Input: part model. Units: mm. Frame: model coordinates. Face numbers are marked on the shaded views. A direction names the side the tool comes from. Give positions to 0.01 mm unless a question says otherwise; leave off trailing zeros. Write each loop counter-clockwise with the first axis right and the second up, starting at its lowest first coordinate (ties: lowest second). Pieces come first, ordered by that corner, then holes. Notation, with made-up numbers: (-23.5, -36) - (-3.5, -36) arc R15 cw to (-3.5, -18) - close; hole circle Ø8 at (-2, 4.25). An arc over 180 degrees is marked (long way). Answer as CSV lines item,"result". Start each with the question number.
Autodesk Inventor part; units mm, degrees
ref_plane "YZ Plane" through (0, 0, 0) normal (1, 0, 0) x (0, 1, 0)
ref_plane "XZ Plane" through (0, 0, 0) normal (0, 1, 0) x (-1, 0, 0)
ref_plane "XY Plane" through (0, 0, 0) normal (0, 0, 1) x (1, 0, 0)
sketch "Sketch1" plane through (0, 0, 0) normal (0, 0, 1) x (1, 0, 0)
  arc A0 (-3.75, -2.5) -> (-3.75, -5) centre (-3.75, -3.75) ccw
  arc A1 (3.75, -5) -> (3.75, -2.5) centre (3.75, -3.75) ccw
  line L0 (-3.75, -2.5) -> (3.75, -2.5)
  line L1 (3.75, -5) -> (-3.75, -5)
  circle A2 centre (-3.75, -3.75) radius 0.75
  circle A3 centre (3.75, -3.75) radius 0.5
  circle A4 centre (3.75, -3.75) radius 0.5
  point P0 (0, 0)
  dimension "d0" = 2.5
  dimension "d1" = 5
  dimension "d4" = 7.5
  dimension "d5" = 3.75
  dimension "d6" = 1.5
  dimension "d7" = 1
  dimension "d77" = 1
extrude "Extrusion1" add sketch "Sketch1" along normal blind 20
sketch "Sketch3" plane through (0, 0, 0) normal (0, 1, 0) x (-1, 0, 0)
  line L0 (5, 0) -> (3.75, 0)
  line L1 (-3.75, 0) -> (3.75, 0)
  line L2 (5, 16.9) -> (2.5, 16.9)
  line L3 (2.5, 16.9) -> (2.5, 20)
  line L4 (2.5, 20) -> (5, 20)
  line L5 (5, 20) -> (5, 16.9)
  line L6 (5, 14.3) -> (2.5, 14.3)
  line L7 (2.5, 14.3) -> (2.5, 11.3)
  line L8 (2.5, 11.3) -> (5, 11.3)
  line L9 (5, 11.3) -> (5, 14.3)
  line L10 (5, 5.7) -> (2.5, 5.7)
  line L11 (2.5, 5.7) -> (2.5, 8.7)
  line L12 (2.5, 8.7) -> (5, 8.7)
  line L13 (5, 8.7) -> (5, 5.7)
  line L14 (5, 0) -> (2.5, 0)
  line L15 (2.5, 0) -> (2.5, 3.1)
  line L16 (2.5, 3.1) -> (5, 3.1)
  line L17 (5, 3.1) -> (5, 0)
  line L18 (-2.5, 2.9) -> (-5, 2.9)
  line L19 (-5, 2.9) -> (-5, 5.9)
  line L20 (-5, 5.9) -> (-2.5, 5.9)
  line L21 (-2.5, 5.9) -> (-2.5, 2.9)
  line L22 (-2.5, 8.5) -> (-5, 8.5)
  line L23 (-5, 8.5) -> (-5, 11.5)
  line L24 (-5, 11.5) -> (-2.5, 11.5)
  line L25 (-2.5, 11.5) -> (-2.5, 8.5)
  line L26 (-2.5, 14.1) -> (-5, 14.1)
  line L27 (-5, 14.1) -> (-5, 17.1)
  line L28 (-5, 17.1) -> (-2.5, 17.1)
  line L29 (-2.5, 17.1) -> (-2.5, 14.1)
  point P0 (0, 0)
  point P1 (0, 0)
  point P2 (0, 0)
  point P3 (0, 0)
  point P4 (0, 0)
  point P5 (0, 0)
  point P6 (0, 0)
  point P7 (0, 0)
  point P8 (0, 0)
  dimension "d49" = 2.5
  dimension "d50" = 2.5
  dimension "d52" = 3.1
  dimension "d53" = 3.1
  dimension "d54" = 3
  dimension "d55" = 3
  dimension "d56" = 3
  dimension "d57" = 3
  dimension "d58" = 3
  dimension "d72" = 10
  dimension "d73" = 5
  dimension "d74" = 0
  dimension "d80" = 0.2
  dimension "d81" = 0.2
  dimension "d82" = 0.2
  dimension "d83" = 0.2
  dimension "d84" = 0.2
  dimension "d85" = 0.2
extrude "Extrusion2" cut sketch "Sketch3" against normal blind 20
extrude "Extrusion3" add sketch "Sketch1" along normal blind 20 contours A3
properties part number "chain_link"
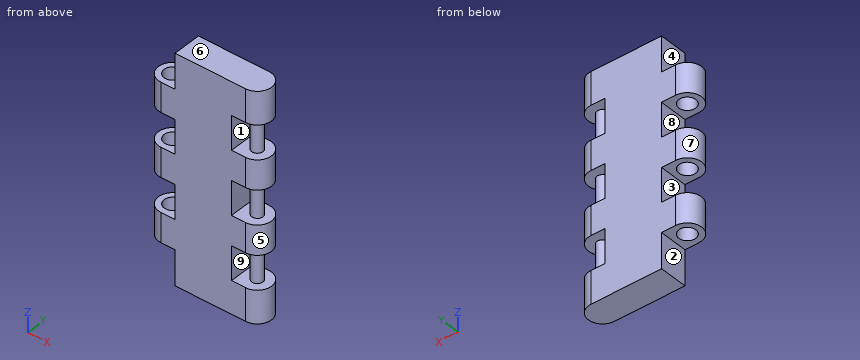
1) Contact query for flat-ended pins moving along their axis: P1, Ø1.2, axis at y = -3.5, z = 4, coming from the +X side; P2, Ø0.8, axis at y = -3.5, z = 13, coming from the -X side; P3, Ø0.8, axis at x = -4, y = -3, coming from the -Z side; P4, Ø1.2, axis at x = 3.5, y = -3.5, coming from the -Z side. Output: stop coordinate, or through.
2) Reachability of the marked faces 1, 2, 3, 4 and 5 from +Z, -Z, +X, -X, +Y, -Y: full face, straight path, thin tool, end or side. Return the list, or none.
3) Cut plane B-B on x = -3.25. Output: boundary loops of the cut face in (y, z).
4) Cut plane A-A on z = 5.25. Output: boundary loops of the cut face in (x, y), and give its area (3 significant figures).
5) Material intervals for line 1 (Z direction, x = -3, y = -4.6); line 2 (X direction, y = -3.75, z = 10.65); line 3 (Y direction, x = -3.75, z = 15.55), sorted ascending. Write a range as from..to.
6) Pull-direction query (Z, two-part tool) for the marked faces 6, 7, 8 and 9; classes: +Z half, -Z half, draft (parallel to the pull), parting line (faces both ways), or undercut.
7) Cut plane C-C on y = -3.75. State how many separate pieces and enclosed holes the cut face has, and give its area (3 significant figures).
Numbers:
1,P1,"stops at x = 4.25"
1,P2,"stops at x = -2.5"
1,P3,"stops at z = 3.1"
1,P4,"stops at z = 0"
2,face 1,"+Y, -Y"
2,face 2,"-Z, -X, +Y, -Y"
2,face 3,"-X, +Y, -Y"
2,face 4,"+Z, -X, +Y, -Y"
2,face 5,"+Z, -Z, +X"
3,outline,"(-5, 3.1) - (-4.31, 3.1) - (-4.31, 5.7) - (-5, 5.7) - close; (-5, 8.7) - (-4.31, 8.7) - (-4.31, 11.3) - (-5, 11.3) - close; (-5, 14.3) - (-4.31, 14.3) - (-4.31, 16.9) - (-5, 16.9) - close; (-3.19, 3.1) - (-2.5, 3.1) - (-2.5, 5.7) - (-3.19, 5.7) - close; (-3.19, 8.7) - (-2.5, 8.7) - (-2.5, 11.3) - (-3.19, 11.3) - close; (-3.19, 14.3) - (-2.5, 14.3) - (-2.5, 16.9) - (-3.19, 16.9) - close"
4,outline,"(-3.75, -5) - (2.5, -5) - (2.5, -2.5) - (-3.75, -2.5) arc R1.25 ccw to start; circle Ø1 at (3.75, -3.75); hole circle Ø1.5 at (-3.75, -3.75)"
4,area,"17.1 mm²"
5,line 1,"z = 3.1..5.7, 8.7..11.3, 14.3..16.9"
5,line 2,"x = -5..-4.5, -3..2.5, 3.25..4.25"
5,line 3,"y = -5..-4.5, -3..-2.5"
6,face 6,"+Z half"
6,face 7,"draft"
6,face 8,"undercut"
6,face 9,"undercut"
7,separate pieces,"4"
7,enclosed holes,"3"
7,area,"144 mm²"
